CAD build for the part. Positions are in the model's coordinates, mm. A direction names the side the tool comes from. Give positions to 0.01 mm unless a question says otherwise; leave off trailing zeros. Write each loop counter-clockwise with the first axis right and the second up, starting at its lowest first coordinate (ties: lowest second). Pieces come first, ordered by that corner, then holes. Notation, with made-up numbers: (-39.75, 34) - (18.25, 34) arc R17 cw to (18.25, 52) - close; hole circle Ø10 at (47, 23.25). An arc over 180 degrees is marked (long way). Write item = value, one per line. Start each with the question number.
Autodesk Inventor part; units mm, degrees
ref_plane "YZ Plane" through (0, 0, 0) normal (1, 0, 0) x (0, 1, 0)
ref_plane "XZ Plane" through (0, 0, 0) normal (0, 1, 0) x (-1, 0, 0)
ref_plane "XY Plane" through (0, 0, 0) normal (0, 0, 1) x (1, 0, 0)
sketch "Sketch1" plane through (0, 0, 0) normal (0, 1, 0) x (-1, 0, 0)
  line L0 (0, 0) -> (25.4, 0)
  line L1 (25.4, 0) -> (25.4, -25.4)
  line L2 (25.4, -25.4) -> (0, -25.4)
  line L3 (0, -25.4) -> (0, 0)
  line L4 (23.8125, -23.8125) -> (23.8125, -1.5875)
  line L5 (23.8125, -1.5875) -> (1.5875, -1.5875)
  line L6 (1.5875, -1.5875) -> (1.5875, -23.8125)
  line L7 (1.5875, -23.8125) -> (23.8125, -23.8125)
  dimension "d0" = 25.4
  dimension "d1" = 25.4
  dimension "d2" = 1.5875
extrude "Extrusion1" add sketch "Sketch1" along normal blind 508
sketch "Sketch2" plane through (0, 0, -25.4) normal (0, 0, -1) x (-1, 0, 0)
  circle A0 centre (12.7, 469.9) radius 6.35
  line L0 (0, 508) -> (25.4, 508)
  point P0 (0, 0)
  dimension "d5" = 12.7
  dimension "d6" = 38.1
extrude "Extrusion2" cut sketch "Sketch2" against normal blind 25.4
sketch "Sketch5" plane through (0, 0, -25.4) normal (0, 0, -1) x (-1, 0, 0)
  circle A0 centre (11.811, 342.9) radius 6.35
  line L0 (25.4, 0) -> (25.4, 508)
  line L1 (25.4, 0) -> (0, 0)
  dimension "d19" = 12.7
  dimension "d20" = 13.589
  dimension "d21" = 342.9
extrude "Extrusion5" cut sketch "Sketch5" against normal blind 25.4
sketch "Sketch6" plane through (0, 0, -25.4) normal (0, 0, -1) x (-1, 0, 0)
  circle A0 centre (12.5567, 405.2777) radius 6.35
  point P0 (0, 0)
  dimension "d24" = 12.7
extrude "Extrusion6" cut sketch "Sketch6" against normal blind 25.4
properties part number "AP 7"
1. Cut at D-D (x = -11.5). Count the separate pieces of the cut face and the enclosed holes in it, then the cut area to 3 significant figures.
2. Wall check: line 1 along Z through (x, y) = (-16.25, 415.5); line 2 along Y through (x, z) = (-12.7, -0.5). Give the ranges that are in metal, low to high.
3. Pin check, flat tip, straight feed: pin 1 Ø1.5 at (y, z) = (280.5, -3) entering from +X. Stop position of the tip, or through.
4. Cut at C-C (y = 172). Give the cut face in (x, z), then the cut area to 3 significant figures.
5. Cut at A-A (y = 469.9). Give the cut face in (x, z).
6. Tool access for faces 1 (the flat face through (-13, 250, -25.4)), 2 (the flat face through (-1.588, 250, -13)): list every direction of +Z, -Z, +X, -X, +Y, -Y with a clear straight run to the whole face (end or side of a thin tool).
7. Cut at B-B (z = -8). Give the cut face in (x, y), then the cut area to 3 significant figures.
8. Mould opens along Y. For faces 3 (the flat face through (-25.4, 250, -13)), 4 (the cylindrical face through (-11.73, 411.574, -0.805)), 5 (the cylindrical face through (-11.9, 476.2, -0.8)), 6 (the flat face through (-1, 508, -13)) say: +Y half, -Y half, draft (parallel to the pull), parting line (faces both ways), or undercut.
Output:
q1.separate_pieces = 8
q1.enclosed_holes = 0
q1.area = 1,490 mm2
q2.line_1 = -25.4 to -23.81, -1.59 to 0
q2.line_2 = 0 to 336.61, 349.19 to 398.93, 411.63 to 463.55, 476.25 to 508
q3.pin_1 = 0
q4.outline = (-25.4, -25.4) - (0, -25.4) - (0, 0) - (-25.4, 0) - close; hole (-23.81, -23.81) - (-1.59, -23.81) - (-1.59, -1.59) - (-23.81, -1.59) - close
q4.area = 151 mm2
q5.outline = (-25.4, -25.4) - (-19.05, -25.4) - (-19.05, -23.81) - (-23.81, -23.81) - (-23.81, -1.59) - (-19.05, -1.59) - (-19.05, 0) - (-25.4, 0) - close; (-6.35, -25.4) - (0, -25.4) - (0, 0) - (-6.35, 0) - (-6.35, -1.59) - (-1.59, -1.59) - (-1.59, -23.81) - (-6.35, -23.81) - close
q6.face_1 = -Z, +X, -X, +Y, -Y
q6.face_2 = +Y, -Y
q7.outline = (-25.4, 0) - (-23.81, 0) - (-23.81, 508) - (-25.4, 508) - close; (-1.59, 0) - (0, 0) - (0, 508) - (-1.59, 508) - close
q7.area = 1,610 mm2
q8.face_3 = draft
q8.face_4 = undercut
q8.face_5 = undercut
q8.face_6 = +Y half
